Work out the finished part from the listing and answer in its coordinate system (mm). A direction names the side the tool comes from. Give positions to 0.01 mm unless a question says otherwise; leave off trailing zeros. Loops run counter-clockwise (first coordinate to the right, second up) from the corner with the lowest first, then second, coordinate; pieces in that order, holes last. Notation, with made-up numbers: (3, -8.5) -> (54, -8.5) arc R16 cw to (54, 3.5) -> close; hole circle Ø9 at (39, -19). An arc over 180 degrees is marked (long way). Answer as CSV lines item,"result". Start each with the question number.
1. Flat-ended cylindrical pins translate along their axes: pin 1 Ø5.5 at (x, z) = (11.5, 3.5) entering from -Y; pin 2 Ø5.5 at (x, y) = (0, 0) entering from -Z; pin 3 Ø1 at (x, y) = (1.5, 0.5) entering from +Z. Find the tip coordinate at first contact, or state that the pin passes through.
2. Find section A-A, the plane z = -2.5. Give the vertices of the cut face in (x, y), and give its area (3 significant figures).
3. Find the intervals of material crossed by line 1 along Y through (x, z) = (0, -18); line 2 along X through (y, z) = (0, -2.9); line 3 along Y through (x, z) = (0, -2.25), in increasing order.
4. Find section D-D, the plane z = -21.5. Give the vertices of the cut face in (x, y).
5. Find section B-B, the plane y = 0. Give the vertices of the cut face in (x, z), and give its area (3 significant figures).
6. A tool of negligible diameter and unlimited length cuts with its end or side. For faces 5 (the face through (0, 0, -4.2)), 6 (the face through (10, 0, 2)), 7 (the face through (-12, 2.5, 2)), 8 (the face through (12, -2.5, 2)), from which of +Z, -Z, +X, -X, +Y, -Y can it reach the whole face along a straight path? Write none if from no direction.
7. Determine the mould class of faces 1 (the face through (13, -9, -12)), 2 (the face through (-0.2, 9.5, -24.5)), 3 (the face through (-14, 8, -12)), 4 (the face through (3, -2, 0)) for opening direction X: +X half, -X half, draft (parallel to the pull), parting line (faces both ways), or undercut.
8. Find section C-C, the plane x = 0. Give the vertices of the cut face in (y, z).
Autodesk Fusion 360 part; units mm, degrees
sketch "Szkic1" plane through (0, 0, 0) normal (0, 0, 1) x (1, 0, 0)
  line L0 (-15, 10) -> (15, 10)
  line L1 (15, 10) -> (15, -10)
  line L2 (15, -10) -> (-15, -10)
  line L3 (-15, -10) -> (-15, 10)
  circle A0 centre (0, 0) radius 3
  circle A1 centre (0, 0) radius 5.5
  line L4 (-15, 2.5) -> (-15, -2.5)
  line L5 (-15, -2.5) -> (15, -2.5)
  line L6 (15, -2.5) -> (15, 2.5)
  line L7 (15, 2.5) -> (-15, 2.5)
  line L8 (-10, 2.5) -> (10, 2.5)
  line L9 (10, 2.5) -> (10, -2.5)
  line L10 (10, -2.5) -> (-10, -2.5)
  line L11 (-10, -2.5) -> (-10, 2.5)
  dimension "d1" = 6
  dimension "d2" = 11
extrude "Wyciągnięcie proste1" add sketch "Szkic1" against normal blind 25 contours L0 L1 L3 A1 L7 L8 | L3 L4 L5 L7 L11 | L1 L5 L6 L7 L9 | L1 L2 L3 A1 L5 L10 | A1 L5 L7 L8 L10 L11 | A1 L5 L7 L8 L9 L10
extrude "Wyciągnięcie proste2" add sketch "Szkic1" against normal blind 4.2 contours A0 A1 L5 L7 L8 L10 | A0 A1 L7 L8 | A0 A1 L5 L7 L8 L10 | A0 A1 L5 L10 | A0 L5 L7 L8 L10 | A0 L7 L8 | A0 L5 L10
extrude "Wyciągnięcie proste3" cut sketch "Szkic1" against normal blind 4 contours A0 L5 L7 L8 L10 | A0 L7 L8 | A0 L5 L10
extrude "Wyciągnięcie proste4" add sketch "Szkic1" along normal blind 5 contours L3 L4 L5 L7 L11 | L1 L5 L6 L7 L9
chamfer "Fazowanie1" distance 3 angle 45 4 edges at (15, -10, -12.5) (15, 10, -12.5) (-15, -10, -12.5) (-15, 10, -12.5)
chamfer "Fazowanie2" distance 1 angle 45 1 faces at (11.8333, 0, -25)
delete_face "Usuń powierzchnię1" 1 faces at (6.159, 0.3074, -24.6667)
Resolved:
1,pin 1,"stops at y = -2.5"
1,pin 2,"stops at z = -4.2"
1,pin 3,"stops at z = -4"
2,outline,"(-15, -7) -> (-12, -10) -> (12, -10) -> (15, -7) -> (15, 7) -> (12, 10) -> (-12, 10) -> (-15, 7) -> close; hole circle Ø6 at (0, 0)"
2,area,"554 mm^2"
3,line 1,"y = -10 to -5.5, 5.5 to 10"
3,line 2,"x = -15 to -3, 3 to 15"
3,line 3,"y = -10 to -3, 3 to 10"
4,outline,"(-15, -7) -> (-12, -10) -> (12, -10) -> (15, -7) -> (15, 7) -> (12, 10) -> (-12, 10) -> (-15, 7) -> close; hole circle Ø11 at (0, 0)"
5,outline,"(-15, -24) -> (-14, -25) -> (-5.5, -25) -> (-5.5, -4.2) -> (5.5, -4.2) -> (5.5, -25) -> (14, -25) -> (15, -24) -> (15, 5) -> (10, 5) -> (10, 0) -> (3, 0) -> (3, -4) -> (-3, -4) -> (-3, 0) -> (-10, 0) -> (-10, 5) -> (-15, 5) -> close"
5,area,"546 mm^2"
6,face 5,"-Z"
6,face 6,"+Z, +Y, -Y"
6,face 7,"+Z, +X, -X, +Y"
6,face 8,"+Z, +X, -X, -Y"
7,face 1,"+X half"
7,face 2,"draft"
7,face 3,"-X half"
7,face 4,"undercut"
8,outline,"(-10, -24) -> (-9, -25) -> (-5.5, -25) -> (-5.5, -4.2) -> (5.5, -4.2) -> (5.5, -25) -> (9, -25) -> (10, -24) -> (10, 0) -> (3, 0) -> (3, -4) -> (-3, -4) -> (-3, 0) -> (-10, 0) -> close"
